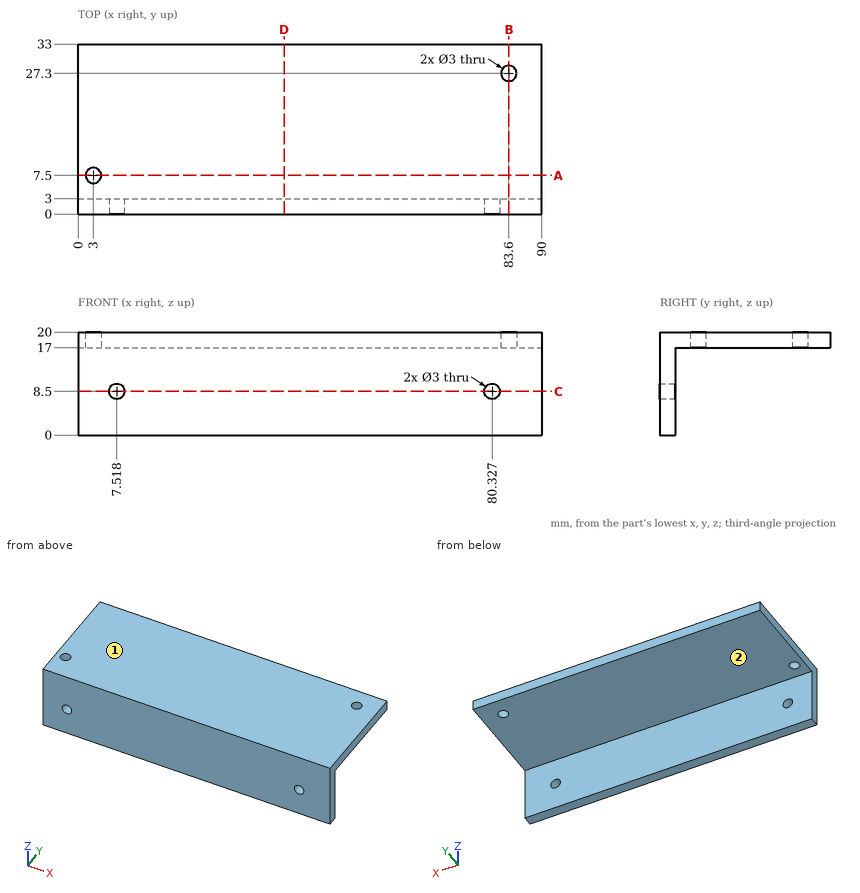
Answer from the drawing. Dimensions are ordinates in mm from the lowest x, y and z of the part. A direction names the side the tool comes from. Round coordinates to 2 decimals unless told otherwise and drop trailing zeros. Write each loop counter-clockwise with the first axis right and the second up, starting at its lowest first coordinate (ties: lowest second). Pieces come first, ordered by that corner, then holes.
1. The part is cut by section C-C, the plane z = 8.5. Determine the outline of the cut face in (x, y), then the cut area to 3 significant figures.
2. Given pin 1 Ø4 at (x, z) = (80.33, 8.5) entering from +Y; pin 2 Ø5 at (x, y) = (83.6, 27.3) entering from -Z, each flat-ended and moving along its own axis, determine where each tip first touches the part or whether it passes through.
3. Straight lines are drawn through the part: L1, parallel to X at y = 0.6, z = 8.5; L2, parallel to Y at x = 3, z = 18.4; L3, parallel to Y at x = 83.6, z = 18.45. For each, find the intervals that lie inside material, in ascending order.
4. The part is cut by section B-B, the plane x = 83.6. Determine the outline of the cut face in (y, z), then the cut area to 3 significant figures.
5. Which of the six approach directions +Z, -Z, +X, -X, +Y, -Y give full straight-line access (tool end or side, diameter ignored) to the marked faces 1 and 2?
6. The part is cut by section A-A, the plane y = 7.5. Determine the outline of the cut face in (x, z), then the cut area to 3 significant figures.
7. The part is cut by section D-D, the plane x = 40. Determine the outline of the cut face in (y, z), then the cut area to 3 significant figures.
Values:
1. outline: (0, 0) - (6.02, 0) - (6.02, 3) - (0, 3) - close; (9.02, 0) - (78.83, 0) - (78.83, 3) - (9.02, 3) - close; (81.83, 0) - (90, 0) - (90, 3) - (81.83, 3) - close
1. area: 252 mm2
2. pin 1: stops at y = 3
2. pin 2: stops at z = 17
3. L1: x = 0 to 6.02, 9.02 to 78.83, 81.83 to 90
3. L2: y = 0 to 6, 9 to 33
3. L3: y = 0 to 25.8, 28.8 to 33
4. outline: (0, 0) - (3, 0) - (3, 17) - (25.8, 17) - (25.8, 20) - (0, 20) - close; (28.8, 17) - (33, 17) - (33, 20) - (28.8, 20) - close
4. area: 141 mm2
5. face 1: +Z, +X, -X, +Y, -Y
5. face 2: -Z, +X, -X, +Y
6. outline: (0, 17) - (1.5, 17) - (1.5, 20) - (0, 20) - close; (4.5, 17) - (90, 17) - (90, 20) - (4.5, 20) - close
6. area: 261 mm2
7. outline: (0, 0) - (3, 0) - (3, 17) - (33, 17) - (33, 20) - (0, 20) - close
7. area: 150 mm2
